from build123d import *

# Parameters (mm, degrees)
SKETCH1_R               = 55
SKETCH1_R_2             = 37.5
BOSS_EXTRUDE1_DEPTH     = 120
CUT_EXTRUDE1_DEPTH      = 144.003496461
CUT_EXTRUDE1_DEPTH_BACK = 144.003496461
SKETCH2_W               = 22
SKETCH2_H               = 14


with BuildPart() as part:
    # Sketch1 → Boss-Extrude1 (new body)
    with BuildSketch(Plane.XY):
        Circle(SKETCH1_R)
        Circle(SKETCH1_R_2, mode=Mode.SUBTRACT)
    extrude(amount=BOSS_EXTRUDE1_DEPTH)

    # Sketch2 → Cut-Extrude1 (cut, two sides: drawn at the far end of the back side and taken through both)
    with BuildSketch(Plane.XY.offset(120).offset(-CUT_EXTRUDE1_DEPTH_BACK)):
        with Locations((0, 37.5)):
            Rectangle(SKETCH2_W, SKETCH2_H)
    extrude(amount=CUT_EXTRUDE1_DEPTH + CUT_EXTRUDE1_DEPTH_BACK, mode=Mode.SUBTRACT)


solid = part.part
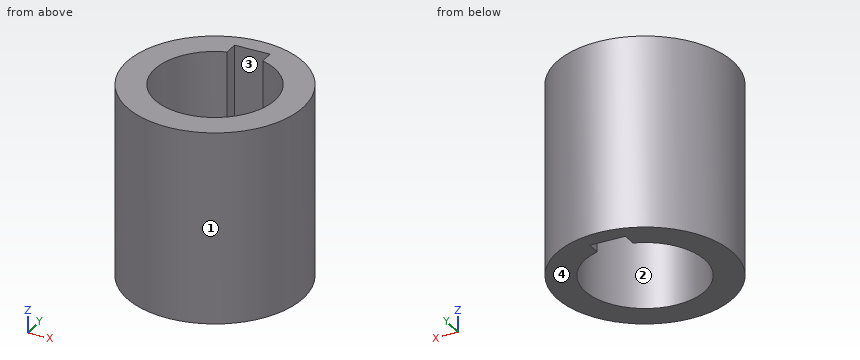
Part model, mm, in its own coordinate system. Face numbers are marked on the shaded views. Give positions to 0.01 mm unless a question says otherwise; leave off trailing zeros. Loops run counter-clockwise (first coordinate to the right, second up) from the corner with the lowest first, then second, coordinate; pieces in that order, holes last. Notation, with made-up numbers: (62.25, 76) -> (66.25, 76) arc R11 cw to (66.25, 90) -> close; hole circle Ø2 at (74.25, -7). An arc over 180 degrees is marked (long way). Write each question's results on one line, items separated by ' | '. Start each with the question number.
Q1. Band-saw the part on A-A on y = 0. List the corners of the cut face in (x, z).
Q2. Band-saw the part on C-C on z = 39.5. List the corners of the cut face in (x, y).
Q3. Pin check, flat tips, straight feed: P1, Ø10, axis at x = -14, z = 84.5, coming from the -Y side; P2, Ø4.5, axis at y = 41, z = 78, coming from the -X side; P3, Ø4, axis at y = 23, z = 86, coming from the +X side. Stop position of each tip, or through.
Q4. Band-saw the part on B-B on x = -31. List the corners of the cut face in (y, z).
Q5. Pull direction X, two halves, no side cores. Call the marked faces 1, 2, 3 and 4: +X half, -X half, draft (parallel to the pull), parting line (faces both ways), or undercut.
Q6. Wall check: L1, parallel to Y at x = 0, z = 86; L2, parallel to X at y = -30, z = 61; L3, parallel to X at y = 10, z = 45. Give the ranges that are in metal, low to high.
Q7. Band-saw the part on D-D on y = -47. List the corners of the cut face in (x, z).
Results are:
1) outline: (-55, 0) -> (-37.5, 0) -> (-37.5, 120) -> (-55, 120) -> close; (37.5, 0) -> (55, 0) -> (55, 120) -> (37.5, 120) -> close
2) outline: circle Ø110 at (0, 0); hole (-11, 35.85) arc R37.5 ccw (long way) to (11, 35.85) -> (11, 44.5) -> (-11, 44.5) -> close
3) P1: stops at y = -54.26 | P2: stops at x = -39.03 | P3: stops at x = 50.83
4) outline: (-45.43, 0) -> (-21.1, 0) -> (-21.1, 120) -> (-45.43, 120) -> close; (21.1, 0) -> (45.43, 0) -> (45.43, 120) -> (21.1, 120) -> close
5) face 1: parting line | face 2: undercut | face 3: undercut | face 4: draft
6) L1: y = -55 to -37.5, 44.5 to 55 | L2: x = -46.1 to -22.5, 22.5 to 46.1 | L3: x = -54.08 to -36.14, 36.14 to 54.08
7) outline: (-28.57, 0) -> (28.57, 0) -> (28.57, 120) -> (-28.57, 120) -> close
